Input: part model. Units: mm. Frame: model coordinates. A direction names the side the tool comes from. Coordinates: 2 decimals unless noted, no trailing zeros. Loops run counter-clockwise (first coordinate to the right, second up) from the corner with the lowest first, then second, coordinate; pieces in that order, holes last. Notation, with made-up numbers: M 3.5,-37.75 L 54.5,-37.75 A17 cw 54.5,-21.75 Z; hole C 55.5,3 d7. An arc over 180 degrees is marked long. Use a Markdown table: item, result. Add a question column.
1. Pin query (flat end, axial travel): pin 1 (8 mm diameter, centred on x = 19.05, y = 25.4, fed in from -Z). Return the tip coordinate at first contact, or that it passes through.
2. Section B-B on y = -25.4. Output: boundary loops of the cut face in (x, z).
3. Section C-C on z = 5. State how many separate pieces and enclosed holes the cut face has, then the cut area to 3 significant figures.
4. Section A-A on x = 0. Output: boundary loops of the cut face in (y, z), then the cut area to 3 significant figures.
5. Set-up query: faces 4 (the cylindrical face through (-0.175, 20.636, 3.131)), 5 (the flat face through (-25.4, 0, 3)). Return all of +Z, -Z, +X, -X, +Y, -Y with unobstructed straight access to the full face (end or side cutting, diameter ignored); none if empty.
6. Draft query along X for faces 1 (the flat face through (0, -31.75, 3)), 2 (the flat face through (7.938, 0, 3)), 3 (the flat face through (25.4, 0, 3)). Return one class per face: +X half, -X half, draft (parallel to the pull), parting line (faces both ways), or undercut.
7. Line query: L1, parallel to Y at x = 19.05, z = 4.5; L2, parallel to Y at x = 18, z = 1.25; L3, parallel to X at y = 11.5, z = 4.5. Output: solid intervals per line, ascending. Write a range as [from, to].
8. Section D-D on x = -19.05. Output: boundary loops of the cut face in (y, z), then the cut area to 3 significant figures.
```python
from build123d import *

# Parameters (mm, degrees)
SKETCH1_W           = 50.8
SKETCH1_H           = 63.5
SKETCH1_R           = 2.5527
BOSS_EXTRUDE1_DEPTH = 6.35


with BuildPart() as part:
    # Sketch1 → Boss-Extrude1 (new body)
    with BuildSketch(Plane.XY):
        Rectangle(SKETCH1_W, SKETCH1_H)
        with Locations(Location((-19.05, 25.4, 0), (0, 0, 180))):
            Circle(SKETCH1_R, mode=Mode.SUBTRACT)
        with Locations((19.05, 25.4)):
            Circle(SKETCH1_R, mode=Mode.SUBTRACT)
        with Locations((19.05, -25.4)):
            Circle(SKETCH1_R, mode=Mode.SUBTRACT)
        with Locations(Location((-19.05, -25.4, 0), (0, 0, 180))):
            Circle(SKETCH1_R, mode=Mode.SUBTRACT)
        with BuildLine():
            Line((-7.9375, -12.7), (-7.9375, 12.7))
            ThreePointArc((-7.9375, 12.7), (0, 20.6375), (7.9375, 12.7))
            Line((7.9375, 12.7), (7.9375, -12.7))
            ThreePointArc((7.9375, -12.7), (0, -20.6375), (-7.9375, -12.7))
        make_face(mode=Mode.SUBTRACT)
    extrude(amount=BOSS_EXTRUDE1_DEPTH)


solid = part.part
```
Answers below:
| question | item | result |
|---|---|---|
| 1 | pin 1 | stops at z = 0 |
| 2 | outline | M -25.4,0 L -21.6,0 L -21.6,6.35 L -25.4,6.35 Z; M -16.5,0 L 16.5,0 L 16.5,6.35 L -16.5,6.35 Z; M 21.6,0 L 25.4,0 L 25.4,6.35 L 21.6,6.35 Z |
| 3 | separate pieces | 1 |
| 3 | enclosed holes | 5 |
| 3 | area | 2,540 mm² |
| 4 | outline | M -31.75,0 L -20.64,0 L -20.64,6.35 L -31.75,6.35 Z; M 20.64,0 L 31.75,0 L 31.75,6.35 L 20.64,6.35 Z |
| 4 | area | 141 mm² |
| 5 | face 4 | +Z, -Z |
| 5 | face 5 | +Z, -Z, -X, +Y, -Y |
| 6 | face 1 | draft |
| 6 | face 2 | undercut |
| 6 | face 3 | +X half |
| 7 | L1 | y = [-31.75, -27.95], [-22.85, 22.85], [27.95, 31.75] |
| 7 | L2 | y = [-31.75, -27.73], [-23.07, 23.07], [27.73, 31.75] |
| 7 | L3 | x = [-25.4, -7.94], [7.94, 25.4] |
| 8 | outline | M -31.75,0 L -27.95,0 L -27.95,6.35 L -31.75,6.35 Z; M -22.85,0 L 22.85,0 L 22.85,6.35 L -22.85,6.35 Z; M 27.95,0 L 31.75,0 L 31.75,6.35 L 27.95,6.35 Z |
| 8 | area | 338 mm² |
